The listing builds one solid part. Answer for the finished solid, in the listing's coordinates (mm). A direction names the side the tool comes from. Round coordinates to 2 decimals unless told otherwise and drop trailing zeros. Order: outer loops, then holes, each group sorted by start corner. A loop starts at its lowest first (then second) coordinate and runs counter-clockwise, first axis right, second up. Notation, with made-up numbers: (-5, 64) -> (22, 64) arc R33 cw to (22, 102) -> close; hole circle Ø9 at (63, 36.5). An arc over 180 degrees is marked (long way). Return JSON: item names as keys, results as strings. Group by question number.
(1) Which of the six approach directions +Z, -Z, +X, -X, +Y, -Y give full straight-line access (tool end or side, diameter ignored) to faces 4 (the face through (0, 12.7, 347)), 5 (the face through (0, 0, 0)), 6 (the face through (-23, -7, 365.125))?
(2) Determine the mould class of faces 1 (the face through (0, 0, 317.5)), 2 (the face through (23, -7, 346.075)), 3 (the face through (-5.506, 24.796, 370.823)) for opening direction X: +X half, -X half, draft (parallel to the pull), parting line (faces both ways), or undercut.
(3) The part is cut by section A-A (z = 334.5). Determine the outline of the cut face in (x, y), plus the area to 3 significant figures.
(4) Each of these flat-tipped pins is pushed along its axis until it touches: pin 1 (10 mm diameter, centred on x = -16.5, z = 233, fed in from -Y); pin 2 (12 mm diameter, centred on x = -16.5, z = 226, fed in from -Y); pin 3 (0.8 mm diameter, centred on y = 26.5, z = 229, fed in from +X). Where does it stop, or does it pass through?
(5) The part is cut by section C-C (z = 172.5). Determine the outline of the cut face in (x, y), plus the area to 3 significant figures.
(6) Consider line 1 (Y direction, x = 0, z = -3); line 2 (Z direction, x = 15.5, y = 0.5); line 3 (Z direction, x = 4, y = -10). Determine where each line is inside the solid, lowest interval first. Write a range as [from, to].
(7) The part is cut by section B-B (z = 276.5). Determine the outline of the cut face in (x, y), plus the area to 3 significant figures.
Autodesk Inventor part; units mm, degrees
ref_plane "YZ Plane" through (0, 0, 0) normal (1, 0, 0) x (0, 1, 0)
ref_plane "XZ Plane" through (0, 0, 0) normal (0, 1, 0) x (-1, 0, 0)
ref_plane "XY Plane" through (0, 0, 0) normal (0, 0, 1) x (1, 0, 0)
sketch "Sketch1" plane through (0, 0, 0) normal (0, 0, 1) x (1, 0, 0)
  circle A0 centre (0, 0) radius 25.4
  dimension "d0" = 50.8
extrude "Extrusion1" add sketch "Sketch1" along normal blind 355.6
sketch "Sketch4" plane through (0, 0, 355.6) normal (0, 0, 1) x (1, 0, 0)
  line L0 (31.0854, 16.4706) -> (47.788, 16.4706)
  line L1 (47.788, 16.4706) -> (47.788, 0)
  line L2 (47.788, 0) -> (31.0854, 0)
  line L3 (31.0854, 0) -> (31.0854, 16.4706)
  point P0 (0, 0)
extrude "Extrusion4" add sketch "Sketch4" against normal blind 3.175
sketch "Sketch5" plane through (0, 0, 352.425) normal (0, 0, -1) x (-1, 0, 0)
  circle A0 centre (0, 0) radius 25.4
  circle A1 centre (0, 0) radius 23.8125
  dimension "d19" = 1.5875
extrude "Extrusion5" cut sketch "Sketch5" along normal blind 6.35
sketch "Sketch6" plane through (0, 0, 0) normal (0, 0, -1) x (-1, 0, 0)
  line L0 (29.0417, -43.641) -> (10.5178, -43.641)
  line L1 (10.5178, -43.641) -> (10.5178, -69.3861)
  line L2 (10.5178, -69.3861) -> (29.0417, -69.3861)
  line L3 (29.0417, -69.3861) -> (29.0417, -43.641)
  point P0 (0, 0)
extrude "Extrusion6" add sketch "Sketch6" against normal blind 3.175
sketch "Sketch7" plane through (0, 0, 3.175) normal (0, 0, 1) x (1, 0, 0)
  circle A0 centre (0, 0) radius 25.4
  circle A1 centre (0, 0) radius 23.8125
extrude "Extrusion7" cut sketch "Sketch7" along normal blind 6.35
sketch "Sketch8" plane through (-29.0417, -69.3861, 0) normal (-1, 0, 0) x (0, 0, 1)
  line L0 (0, 0) -> (0, 25.7451)
  line L1 (3.175, 25.7451) -> (3.175, 0)
  line L2 (0, 0) -> (3.175, 0)
  line L3 (3.175, 0) -> (3.175, 25.7451)
  line L4 (3.175, 25.7451) -> (0, 25.7451)
  line L5 (0, 25.7451) -> (0, 0)
  point P0 (0, 69.3861)
extrude "Extrusion8" cut sketch "Sketch8" against normal through all
sketch "Sketch9" plane through (0, 0, 355.6) normal (0, 0, 1) x (1, 0, 0)
  line L0 (31.0854, 16.4706) -> (47.788, 16.4706)
  line L1 (31.0854, 16.4706) -> (47.788, 16.4706)
  line L2 (47.788, 16.4706) -> (47.788, 0)
  line L3 (47.788, 0) -> (31.0854, 0)
  line L4 (31.0854, 0) -> (31.0854, 16.4706)
  point P0 (0, 0)
extrude "Extrusion9" cut sketch "Sketch9" against normal blind 6.35
sketch "Sketch10" plane through (0, 0, 346.075) normal (0, 0, 1) x (1, 0, 0)
  circle A0 centre (0, 0) radius 25.4
  line L0 (2.54, 25.4) -> (2.54, 26.67)
  line L1 (2.54, 26.67) -> (0, 26.67)
  line L2 (0, 26.67) -> (0, 25.4)
  line L3 (-2.54, 25.4) -> (-2.54, 26.67)
  line L4 (-2.54, 26.67) -> (0, 26.67)
  line L5 (0, 26.67) -> (0, 25.4)
  arc A1 (2.54, 25.2727) -> (-2.54, 25.2727) centre (0, 0) ccw
  line L6 (2.54, 25.4) -> (2.54, 25.2727)
  line L7 (-2.54, 25.4) -> (-2.54, 25.2727)
  dimension "d30" = 2.54
  dimension "d31" = 1.27
  dimension "d32" = 2.54
  dimension "d33" = 1.27
extrude "Extrusion10" add sketch "Sketch10" against normal blind 168.275 contours A0 L2 L1 L0 L6 | L7 L3 L4 L2 A0
sketch "Sketch11" plane through (-2.54, 26.67, 346.075) normal (0, 1, 0) x (1, 0, 0)
  line L0 (5.08, 168.275) -> (0, 168.275)
  line L1 (0, 0) -> (0, 168.275)
  line L2 (5.08, 168.275) -> (0, 168.275)
  line L3 (0, 168.275) -> (0, 167.64)
  line L4 (0, 167.64) -> (5.08, 167.64)
  line L5 (5.08, 167.64) -> (5.08, 168.275)
  line L6 (5.08, 168.275) -> (0, 168.275)
  line L7 (0, 168.275) -> (0, 168.91)
  line L8 (0, 168.91) -> (5.08, 168.91)
  line L9 (5.08, 168.91) -> (5.08, 168.275)
  point P0 (2.54, 346.075)
  dimension "d36" = 0.635
  dimension "d37" = 0.635
sketch "Sketch12" plane through (0, 0, 177.8) normal (0, 0, -1) x (-1, 0, 0)
  line L0 (2.54, 26.67) -> (-2.54, 26.67)
  line L1 (-2.54, 26.67) -> (-2.54, 25.2727)
  line L2 (-2.54, 25.2727) -> (2.54, 25.2727)
  line L3 (2.54, 25.2727) -> (2.54, 26.67)
  line L4 (2.54, 26.67) -> (2.54, 25.2727)
  line L5 (-2.54, 26.67) -> (2.54, 26.67)
  arc A0 (2.54, 25.2727) -> (-2.54, 25.2727) centre (0, 0) ccw
  arc A1 (-2.54, 25.2727) -> (2.54, 25.2727) centre (0, 0) ccw
  arc A2 (2.54, 25.2727) -> (-2.54, 25.2727) centre (0, 0) ccw
extrude "Extrusion11" add sketch "Sketch12" along normal blind 0.635 contours L3 A0 L1 L0
extrude "Extrusion12" add sketch "Sketch11" along normal blind 1.27
sketch "Sketch13" plane through (0, 0, 355.6) normal (0, 0, 1) x (1, 0, 0)
  line L0 (13.9466, 0.955) -> (12.6912, 0.4731)
  line L1 (13.8404, 1.9655) -> (13.9466, 0.955)
  circle A0 centre (0, 0) radius 13.9792
  circle A1 centre (0, 0) radius 25.4
  circle A2 centre (0, 0) radius 23.8125
  circle A3 centre (0, 0) radius 23.8125
extrude "Extrusion13" add sketch "Sketch13" along normal blind 9.525 contours A2
sketch "Sketch14" plane through (0, 0, 365.125) normal (0, 0, 1) x (1, 0, 0)
  circle A0 centre (0, 0) radius 25.4
  arc A1 (13.9792, 0) -> (13.9792, 0) centre (0, 0) ccw
  circle A2 centre (0, 0) radius 13.9792
extrude "Extrusion14" add sketch "Sketch14" along normal blind 3.175
sketch "Sketch16" plane through (0, 0, 0) normal (0, 0, -1) x (-1, 0, 0)
  circle A0 centre (0, 0) radius 23.8125
  circle A1 centre (0, 0) radius 13.9792
  point P0 (-13.9792, 0)
  point P1 (-13.9792, 0)
extrude "Extrusion15" add sketch "Sketch16" along normal blind 9.525
sketch "Sketch17" plane through (0, 0, -9.525) normal (0, 0, -1) x (-1, 0, 0)
  circle A0 centre (0, 0) radius 25.4
  line L0 (8.8437, -9.1148) -> (9.2337, -9.3135)
  circle A1 centre (0, 0) radius 13.9792
  point P0 (13.9792, 0)
extrude "Extrusion16" add sketch "Sketch17" along normal blind 3.175
sketch "Sketch18" plane through (-2.54, 26.67, 346.075) normal (0, 1, 0) x (1, 0, 0)
  line L0 (5.08, 168.91) -> (5.08, 0)
  line L1 (0, 0) -> (5.08, 0)
  line L2 (5.08, 0) -> (5.08, 7.62)
  line L3 (5.08, 7.62) -> (0, 7.62)
  line L4 (0, 7.62) -> (0, 0)
  line L5 (0, 167.64) -> (5.08, 167.64)
  line L6 (0, 0) -> (0, 168.91)
  line L7 (5.08, 167.64) -> (0, 167.64)
  line L8 (0, 167.64) -> (0, 160.02)
  line L9 (0, 160.02) -> (5.08, 160.02)
  line L10 (5.08, 160.02) -> (5.08, 167.64)
  point P0 (2.54, 346.075)
  dimension "d50" = 7.62
  dimension "d51" = 7.62
extrude "Extrusion17" cut sketch "Sketch18" against normal blind 1.27 contours L0 L9 L6 L5 | L0 L1 L4 L3
sketch "Sketch19" plane through (0, 0, 368.3) normal (0, 0, 1) x (1, 0, 0)
  circle A0 centre (0, 0) radius 15.0616
extrude "Extrusion18" add sketch "Sketch19" against normal blind 25.4
sketch "Sketch20" plane through (0, 0, 368.3) normal (0, 0, 1) x (1, 0, 0)
  line L0 (0, 0) -> (-25.4, 0)
  circle A0 centre (0, 0) radius 25.4
  arc A1 (-12.6912, 0.4731) -> (-12.6912, -0.4731) centre (0, 0) ccw
  line L1 (-12.7, 0) -> (-12.7, 12.7)
  line L2 (-12.7, 12.7) -> (12.7, 12.7)
  line L3 (12.7, 12.7) -> (12.7, -12.7)
  line L4 (12.7, -12.7) -> (-12.7, -12.7)
  line L5 (-12.7, -12.7) -> (-12.7, 0)
  dimension "d56" = 12.7
  dimension "d57" = 25.4
  dimension "d58" = 25.4
  dimension "d59" = 25.4
extrude "Extrusion19" cut sketch "Sketch20" against normal blind 50.8 contours L1 L2 L3 L4 L5
sketch "Sketch24" plane through (0, 0, 368.3) normal (0, 0, 1) x (1, 0, 0)
  circle A0 centre (0, 0) radius 25.4
  line L0 (12.7, 12.7) -> (12.7, -12.7)
  line L1 (-12.7, -12.7) -> (-12.7, 12.7)
  line L2 (12.7, -12.7) -> (-12.7, -12.7)
  line L3 (-12.7, -12.7) -> (-12.7, 12.7)
  line L4 (-12.7, 12.7) -> (12.7, 12.7)
  line L5 (12.7, 12.7) -> (12.7, -12.7)
extrude "Extrusion24" add sketch "Sketch24" along normal blind 8.382
sketch "Sketch25" plane through (-12.7, -12.7, 317.5) normal (1, 0, 0) x (0, 0, -1)
  line L0 (-47.625, 38.1) -> (-59.182, 38.1)
  line L1 (-53.4035, 38.1) -> (-53.4035, -12.7)
  line L2 (-47.625, -12.7) -> (-59.182, -12.7)
  circle A0 centre (-53.4035, 12.7) radius 2.54
  point P0 (317.5, 12.7)
  dimension "d73" = 5.08
extrude "Extrusion25" cut sketch "Sketch25" against normal blind 8.382
extrude "Extrusion26" cut sketch "Sketch25" along normal blind 50.8
sketch "Sketch26" plane through (-12.7, -12.7, 317.5) normal (1, 0, 0) x (0, 0, -1)
  point P0 (317.5, 12.7)
properties part number "Axel_SBail"
Answer below:
{
 "1": {"face 4": "+Z", "face 5": "-Z", "face 6": "none"},
 "2": {"face 1": "undercut", "face 2": "draft", "face 3": "parting line"},
 "3": {"outline": "(-2.54, 25.27) arc R25.4 ccw (long way) to (2.54, 25.27) -> (2.54, 26.67) -> (-2.54, 26.67) -> close; hole (-12.7, -12.7) -> (12.7, -12.7) -> (12.7, 12.7) -> (-12.7, 12.7) -> close", "area": "1,390 mm²"},
 "4": {"pin 1": "stops at y = -22.65", "pin 2": "stops at y = -23.13", "pin 3": "stops at x = 2.54"},
 "5": {"outline": "circle Ø50.8 at (0, 0)", "area": "2,030 mm²"},
 "6": {"line 1": "y = [-23.81, -13.98], [13.98, 23.81]", "line 2": "z = [-12.7, 368.41], [373.39, 376.68]", "line 3": "z = [0, 317.5]"},
 "7": {"outline": "(-2.54, 25.27) arc R25.4 ccw (long way) to (2.54, 25.27) -> (2.54, 26.67) -> (-2.54, 26.67) -> close", "area": "2,030 mm²"}
}
